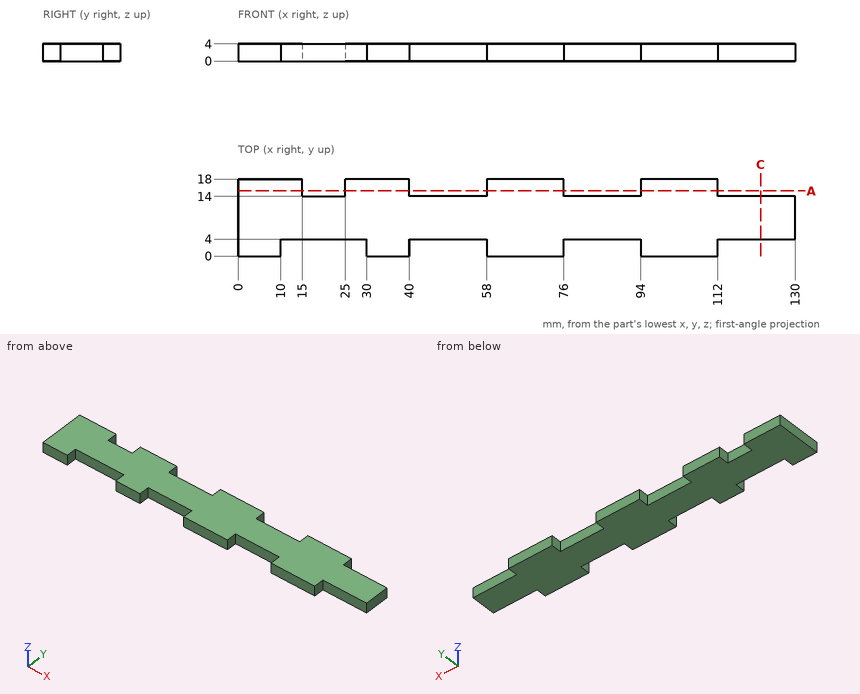
Answer from the drawing. Dimensions are ordinates in mm from the lowest x, y and z of the part. Give positions to 0.01 mm unless a question says otherwise; leave off trailing zeros. Write each loop counter-clockwise with the first axis right and the second up, starting at its lowest first coordinate (ties: lowest second). Pieces come first, ordered by that corner, then holes. Notation, with made-up numbers: (-13, 62) -> (20, 62) arc R19 ccw to (20, 97) -> close; hole circle Ø2 at (38.25, 15). An arc over 180 degrees is marked (long way). One line per question, with ' | ' between items. Start each with the question number.
1. Given pin 1 Ø2 at (y, z) = (17, 1) entering from +X; pin 2 Ø1.2 at (y, z) = (2, 2) entering from -X; pin 3 Ø2 at (x, z) = (89, 2.5) entering from +Y, each flat-ended and moving along its own axis, determine where each tip first touches the part or whether it passes through.
2. Section A-A (y = 15.25) is taken. Determine the outline of the cut face in (x, z), plus the area to 3 significant figures.
3. Find the intervals of material crossed by probe 1 along X at (y, z) = (2.25, 3.05); probe 2 along X at (y, z) = (16.5, 0.6); probe 3 along Y at (x, z) = (26.5, 1.45), in increasing order.
4. Section C-C (x = 122) is taken. Determine the outline of the cut face in (y, z), plus the area to 3 significant figures.
Response values:
1) pin 1: x = 112 | pin 2: x = 0 | pin 3: y = 14
2) outline: (0, 0) -> (15, 0) -> (15, 4) -> (0, 4) -> close; (25, 0) -> (40, 0) -> (40, 4) -> (25, 4) -> close; (58, 0) -> (76, 0) -> (76, 4) -> (58, 4) -> close; (94, 0) -> (112, 0) -> (112, 4) -> (94, 4) -> close | area: 264 mm2
3) probe 1: 0 to 10, 30 to 40, 58 to 76, 94 to 112 | probe 2: 0 to 15, 25 to 40, 58 to 76, 94 to 112 | probe 3: 4 to 18
4) outline: (4, 0) -> (14, 0) -> (14, 4) -> (4, 4) -> close | area: 40.0 mm2
